For this review, take the finished solid that the model builds, in its own axes (mm). Round coordinates to 2 decimals unless told otherwise and drop trailing zeros. Loops run counter-clockwise (first coordinate to the right, second up) from the corner with the lowest first, then second, coordinate; pieces in that order, holes last.
1. Consider section A-A on z = 6. State the section outline as (x, y) points.
2. Consider section C-C on x = -0.9. State the section outline as (y, z) points.
3. Consider section D-D on x = -1.9. State the section outline as (y, z) points, then the cut area to 3 significant figures.
4. Draft analysis for pull direction X (two halves, no side actions). For faces 1 (the cylindrical face through (-1.5, -0.07, 4.93)), 2 (the flat face through (-1.07, -1.88, 4.93)), 3 (the flat face through (1.07, 1.88, 4.93)), state which applies: released by +X, released by -X, zero draft, split by the parting line, or undercut.
5. To check wall thickness, follow line 1 along Y through (x, z) = (0.5, 6.5); line 2 along X through (y, z) = (0.35, 9); line 3 along X through (y, z) = (0.7, 5.25). State the ranges of each line that lie inside material, in increasing order.
6. Consider section B-B on y = 0. State the section outline as (x, z) points, then the cut area to 3 significant figures.
7. Clearance check with flat-ended pins moving along their axes: pin 1 Ø1 at (x, z) = (-1, 2.5) entering from +Y; pin 2 Ø1.5 at (x, z) = (1.5, 2) entering from -Y. State where each tip first meets the part, or that it passes through.
Autodesk Inventor part; units mm, degrees
ref_plane "YZ Plane" through (0, 0, 0) normal (1, 0, 0) x (0, 1, 0)
ref_plane "XZ Plane" through (0, 0, 0) normal (0, 1, 0) x (-1, 0, 0)
ref_plane "XY Plane" through (0, 0, 0) normal (0, 0, 1) x (1, 0, 0)
sketch "Эскиз1" plane through (0, 0, 0) normal (0, 0, 1) x (1, 0, 0)
  circle A0 centre (0, 0) radius 1.5
  circle A1 centre (0, 0) radius 2.5 construction
  line L0 (-2.1651, 1.25) -> (0, 2.5)
  line L1 (0, 2.5) -> (2.1651, 1.25)
  line L2 (2.1651, 1.25) -> (2.1651, -1.25)
  line L3 (2.1651, -1.25) -> (0, -2.5)
  line L4 (0, -2.5) -> (-2.1651, -1.25)
  line L5 (-2.1651, -1.25) -> (-2.1651, 1.25)
  dimension "d1" = 5
  dimension "d0" = 3
extrude "Выдавливание1" add sketch "Эскиз1" along normal blind 10
properties part number "стойка для платы 10мм" material "Латунь, мягкая, желтая"
Resolved:
1. outline: (-2.17, -1.25) - (0, -2.5) - (2.17, -1.25) - (2.17, 1.25) - (0, 2.5) - (-2.17, 1.25) - close; hole circle Ø3 at (0, 0)
2. outline: (-1.98, 0) - (-1.2, 0) - (-1.2, 10) - (-1.98, 10) - close; (1.2, 0) - (1.98, 0) - (1.98, 10) - (1.2, 10) - close
3. outline: (-1.4, 0) - (1.4, 0) - (1.4, 10) - (-1.4, 10) - close
3. area: 28.1 mm2
4. face 1: undercut
4. face 2: released by -X
4. face 3: released by +X
5. line 1: y = -2.21 to -1.41, 1.41 to 2.21
5. line 2: x = -2.17 to -1.46, 1.46 to 2.17
5. line 3: x = -2.17 to -1.33, 1.33 to 2.17
6. outline: (-2.17, 0) - (-1.5, 0) - (-1.5, 10) - (-2.17, 10) - close; (1.5, 0) - (2.17, 0) - (2.17, 10) - (1.5, 10) - close
6. area: 13.3 mm2
7. pin 1: stops at y = 2.21
7. pin 2: stops at y = -2.07
